from build123d import *

# Parameters (mm, degrees)
SKETCH2_W           = 127
SKETCH2_H           = 406.4
BOSS_EXTRUDE1_DEPTH = 3.175
SKETCH3_W           = 127
SKETCH3_H           = 3.175
BOSS_EXTRUDE2_DEPTH = 76.2
FILLET1_R           = 3.175
FILLET2_R           = 6.35
SKETCH4_R           = 6.35
SKETCH4_R_2         = 2.54
CUT_EXTRUDE1_DEPTH  = 416.840163104
SKETCH5_R           = 2.15
SKETCH5_R_2         = 4.7625
CUT_EXTRUDE2_DEPTH  = 227.117071448


with BuildPart() as part:
    # Sketch2 → Boss-Extrude1 (new body)
    with BuildSketch(Plane.XY):
        Rectangle(SKETCH2_W, SKETCH2_H)
    extrude(amount=BOSS_EXTRUDE1_DEPTH)

    # Sketch3 → Boss-Extrude2 (add)
    with BuildSketch(Plane.XY.offset(3.175)):
        with Locations((0, -201.6125)):
            Rectangle(SKETCH3_W, SKETCH3_H)
    extrude(amount=BOSS_EXTRUDE2_DEPTH)

    # Fillet1
    fillet1_edges = [part.edges().sort_by_distance(p)[0] for p in [
        (0, -200.025, 3.175),
        (0, -203.2, 0),
    ]]
    fillet(fillet1_edges, radius=FILLET1_R)

    # Fillet2
    fillet2_edges = [part.edges().sort_by_distance(p)[0] for p in [
        (-63.5, -201.6125, 79.375),
        (63.5, -201.6125, 79.375),
        (-63.5, 203.2, 1.5875),
        (63.5, 203.2, 1.5875),
    ]]
    fillet(fillet2_edges, radius=FILLET2_R)

    # Sketch4 → Cut-Extrude1 (cut, through all)
    with BuildSketch(Plane(origin=(0, -200.025, 0), x_dir=(1, 0, 0), z_dir=(0, 1, 0))):
        with Locations(Location((-9.525, -33.175, 0), (0, 0, 270))):
            Circle(SKETCH4_R)
        with Locations(Location((-39.6875, -15.7125, 0), (0, 0, 270))):
            Circle(SKETCH4_R_2)
        with Locations(Location((-39.6875, -50.6375, 0), (0, 0, 270))):
            Circle(SKETCH4_R_2)
        with Locations(Location((39.6875, -15.7125, 0), (0, 0, 270))):
            Circle(SKETCH4_R_2)
        with Locations(Location((39.6875, -50.6375, 0), (0, 0, 270))):
            Circle(SKETCH4_R_2)
    extrude(amount=-CUT_EXTRUDE1_DEPTH, mode=Mode.SUBTRACT)

    # Sketch5 → Cut-Extrude2 (cut, through all)
    with BuildSketch(Plane.XY.offset(3.175)):
        with Locations((10.273, 76.475)):
            Circle(SKETCH5_R)
        with Locations((40.273, 76.475)):
            Circle(SKETCH5_R)
        with Locations((40.273, 106.175)):
            Circle(SKETCH5_R)
        with Locations((10.273, 106.175)):
            Circle(SKETCH5_R)
        with Locations((-38.1, 187.96)):
            Circle(SKETCH5_R_2)
        with Locations((38.1, 187.96)):
            Circle(SKETCH5_R_2)
        with Locations((-38.1, -165.1)):
            Circle(SKETCH5_R_2)
        with Locations((38.1, -165.1)):
            Circle(SKETCH5_R_2)
    extrude(amount=-CUT_EXTRUDE2_DEPTH, mode=Mode.SUBTRACT)


solid = part.part
Here's how the part is built. I have some questions about the finished solid (model axes, mm). A direction names the side the tool comes from. Coordinates: 2 decimals unless noted, no trailing zeros. Order: outer loops, then holes, each group sorted by start corner. A loop starts at its lowest first (then second) coordinate and runs counter-clockwise, first axis right, second up. Notation, with made-up numbers: M 41.25,39 L 73.25,39 A21 ccw 73.25,50 Z; hole C 41,70 d6. An arc over 180 degrees is marked long. Answer as CSV lines item,"result". Start each with the question number.
1. I need wall thicknesses on line 1 (Z direction, x = 40.5, y = 48) (3 decimals); line 2 (Y direction, x = -38, z = 2); line 3 (Y direction, x = 18.5, z = 7.5) (3 decimals). Which ranges of each line are inside material? Lowest first, please. Write a range as [from, to].
2. I want a section at D-D, the plane y = 7.5. Write out the boundary of the cut face in (x, z) (3 decimals).
3. I want a section at A-A, the plane y = 187.96. Write out the boundary of the cut face in (x, z) (1 decimal), and give its area (3 significant figures).
4. For pin 1 (4 mm diameter, centred on x = 42.5, y = 53, fed in from +Z) (3 decimals); pin 2 (6.5 mm diameter, centred on x = 39.69, z = 50.64, fed in from +Y) (3 decimals), each with a flat end and sliding along its axis, tell me the tip position at first contact or that it passes through.
5. On a 3-axis mill with a long thin cutter (end or side, diameter ignored), from which of +Z, -Z, +X, -X, +Y, -Y can I reach the whole of each face in a straight line? I mean faces 5 (the flat face through (-1, 6, 3.175)), 6 (the cylindrical face through (40.298, -169.325, 1.61)). Say none if no direction works.
6. I want a section at C-C, the plane x = 16. Write out the boundary of the cut face in (y, z) (3 decimals), and give its area (3 significant figures).
7. I want a section at B-B, the plane z = 35. Write out the boundary of the cut face in (x, y) (3 decimals), and give its area (3 significant figures).
8. We'd pull the mould along Y, two halves only. Please class faces 1 (the flat face through (-1, -200.025, 42)), 2 (the cylindrical face through (-38.72, 192.68, 1.61)), 3 (the flat face through (-63.5, -4, 1)), 4 (the cylindrical face through (-39.13, -169.75, 1.61)): released by +Y, released by -Y, zero draft, split by the parting line, or undercut.
Recorded:
1,line 1,"z = [0, 3.175]"
1,line 2,"y = [-202.97, -169.86], [-160.34, 183.2], [192.72, 203.2]"
1,line 3,"y = [-203.2, -200.025]"
2,outline,"M -63.5,0 L 63.5,0 L 63.5,3.175 L -63.5,3.175 Z"
3,outline,"M -63.5,0 L -42.9,0 L -42.9,3.2 L -63.5,3.2 Z; M -33.3,0 L 33.3,0 L 33.3,3.2 L -33.3,3.2 Z; M 42.9,0 L 63.5,0 L 63.5,3.2 L 42.9,3.2 Z"
3,area,"343 mm2"
4,pin 1,"stops at z = 3.175"
4,pin 2,"stops at y = -200.025"
5,face 5,"+Z, +X, -X, +Y"
5,face 6,"+Z, -Z"
6,outline,"M -203.2,3.175 A3.175 ccw -200.025,0 L 203.2,0 L 203.2,3.175 L -196.85,3.175 A3.175 cw -200.025,6.35 L -200.025,79.375 L -203.2,79.375 Z"
6,area,"1,530 mm2"
7,outline,"M -63.5,-203.2 L -15.607,-203.2 L -15.607,-200.025 L -63.5,-200.025 Z; M -3.443,-203.2 L 63.5,-203.2 L 63.5,-200.025 L -3.443,-200.025 Z"
7,area,"365 mm2"
8,face 1,"released by +Y"
8,face 2,"undercut"
8,face 3,"zero draft"
8,face 4,"undercut"
